Could you check a few things on this model? Use its own coordinates, in mm. A direction names the side the tool comes from. Coordinates: 2 decimals unless noted, no trailing zeros. Order: outer loops, then holes, each group sorted by start corner. A loop starts at its lowest first (then second) coordinate and runs counter-clockwise, first axis right, second up. Notation, with made-up numbers: (88.25, 1.5) -> (117.25, 1.5) arc R18 cw to (117.25, 26.5) -> close; hole circle Ø1 at (11.5, -31). An arc over 180 degrees is marked (long way). Put each result on its own line as item: value. Start each with the question number.
Q1. Will these pins go through, and if not, where does the flat tip stop? pin 1 (5 mm diameter, centred on x = -19, y = 8.5, fed in from +Z); pin 2 (8 mm diameter, centred on x = 20.5, y = 41.5, fed in from -Z); pin 3 (2.5 mm diameter, centred on x = -7.5, y = 60, fed in from +Z).
Q2. For faces 1 (the face through (18, 45, 25)), 2 (the face through (-0.6, 2, 9.2)), 3 (the face through (-18, 45, 25)), which set-ups out of +Z, -Z, +X, -X, +Y, -Y let a thin tool reach every point of the face, with its end or its side?
Q3. We'd pull the mould along Y, two halves only. Please class faces 4 (the face through (0, 48, 20)), 5 (the face through (-14.418, 10.058, -45.783)), 6 (the face through (21.01, 22.85, 25.04)): +Y half, -Y half, draft (parallel to the pull), parting line (faces both ways), or undercut.
Q4. Please list where these lines run through material, in increasing order: line 1 along Y through (x, z) = (17.5, -14.5); line 2 along Z through (x, y) = (-31, 4.5); line 3 along X through (y, z) = (16, -6).
Q5. If we section it at A-A (y = 48): Please give me the cut outline in (x, z), and give its area (3 significant figures).
from build123d import *

# Parameters (mm, degrees)
SKETCH2_R           = 1.15
SKETCH2_R_2         = 5
CUT_EXTRUDE1_DEPTH  = 74.484692283
BOSS_EXTRUDE1_START = 20
SKETCH6_R           = 5
SKETCH6_R_2         = 1
BOSS_EXTRUDE1_DEPTH = 10
FILLET1_R           = 10
CHAMFER1_SIZE       = 2


with BuildPart() as part:
    # Sketch1 → Revolve1 (revolve)
    with BuildSketch(Plane.XY, mode=Mode.PRIVATE) as revolve1_sk:
        Polygon((45, 0), (50, 5), (50, 15), (45, 20), (5, 20), (5, 0), align=None)
        Polygon((9, 2), (44.171572875, 2), (48, 5.828427125), (48, 14.171572875), (44.171572875, 18), (9, 18), align=None, mode=Mode.SUBTRACT)
    revolve(revolve1_sk.sketch.rotate(Axis((0, -3.9, 0), (0, 1, 0)), 90), axis=Axis((0, -3.9, 0), (0, 1, 0)))

    # Sketch2 → Cut-Extrude1 (cut, through all)
    with BuildSketch(Plane.XZ):
        with Locations(Location((7.5, 0, 0), (0, 0, 270))):
            Circle(SKETCH2_R)
        with Locations(Location((0, 7.5, 0), (0, 0, 270))):
            Circle(SKETCH2_R)
        with Locations(Location((-7.5, 0, 0), (0, 0, 270))):
            Circle(SKETCH2_R)
        with Locations(Location((0, -7.5, 0), (0, 0, 270))):
            Circle(SKETCH2_R)
        with Locations(Location((0, 0, 0), (0, 0, 270))):
            Circle(SKETCH2_R_2)
    extrude(amount=-CUT_EXTRUDE1_DEPTH, mode=Mode.SUBTRACT)

    # Sketch6 → Boss-Extrude1 (add)
    with BuildSketch(Plane.XY.offset(BOSS_EXTRUDE1_START)):
        with BuildLine():
            Line((18, 60), (18, 20))
            Line((18, 20), (-18, 20))
            Line((-18, 20), (-18, 60))
            ThreePointArc((-18, 60), (0, 78), (18, 60))
        make_face()
        with Locations((0, 60)):
            Circle(SKETCH6_R, mode=Mode.SUBTRACT)
        with Locations((0, 52.5)):
            Circle(SKETCH6_R_2, mode=Mode.SUBTRACT)
        with Locations((7.5, 60)):
            Circle(SKETCH6_R_2, mode=Mode.SUBTRACT)
        with Locations((0, 67.5)):
            Circle(SKETCH6_R_2, mode=Mode.SUBTRACT)
        with Locations((-7.5, 60)):
            Circle(SKETCH6_R_2, mode=Mode.SUBTRACT)
    extrude(amount=BOSS_EXTRUDE1_DEPTH)

    # Fillet1
    fillet1_edges = [part.edges().sort_by_distance(p)[0] for p in [
        (-18, 20, 25),
        (18, 20, 25),
    ]]
    fillet(fillet1_edges, radius=FILLET1_R)

    # Chamfer1
    # the kernel refuses this chamfer: 2 mm, written as the material it takes off along each edge
    with BuildSketch(Plane(origin=(0, 60, 30), x_dir=(-1, 0, 0), z_dir=(0, -1, 0))) as chamfer1_piece_1:
        Polygon((18, CHAMFER1_SIZE), (18 - CHAMFER1_SIZE, 0), (18, 0), align=None)
    revolve(axis=Axis((0, 60, 30), (0, 0, -1)), revolution_arc=180, mode=Mode.SUBTRACT)
    with BuildSketch(Plane(origin=(-18, 30, 30), x_dir=(-0.027495876610585647, 0, -0.9996219169112968), z_dir=(0, 1, 0)), Plane(origin=(18, 60, 30), x_dir=(0.027495876610585647, 0, -0.9996219169112968), z_dir=(0, -1, 0))) as chamfer1_piece_2:
        Polygon((CHAMFER1_SIZE * 0.999621916911, -CHAMFER1_SIZE * 0.0274958766106), (-CHAMFER1_SIZE * 0.0274958766106, -CHAMFER1_SIZE * 0.999621916911), (0, 0), align=None)
    extrude(amount=30, mode=Mode.SUBTRACT)
    with BuildSketch(Plane(origin=(0, 60, 20), x_dir=(-1, 0, 0), z_dir=(0, -1, 0))) as chamfer1_piece_3:
        Polygon((18, -CHAMFER1_SIZE), (18 - CHAMFER1_SIZE, 0), (18, 0), align=None)
    revolve(axis=Axis((0, 60, 20), (0, 0, -1)), revolution_arc=180, mode=Mode.SUBTRACT)
    with BuildSketch(Plane(origin=(-18, 30, 20), x_dir=(-0.027495876610585647, 0, 0.9996219169112968), z_dir=(0, 1, 0)), Plane(origin=(18, 60, 20), x_dir=(0.027495876610585647, 0, 0.9996219169112968), z_dir=(0, -1, 0))) as chamfer1_piece_4:
        Polygon((CHAMFER1_SIZE * 0.999621916911, CHAMFER1_SIZE * 0.0274958766106), (-CHAMFER1_SIZE * 0.0274958766106, CHAMFER1_SIZE * 0.999621916911), (0, 0), align=None)
    extrude(amount=30, mode=Mode.SUBTRACT)
    with BuildSketch(Plane(origin=(-28, 30, 20), x_dir=(-0.49213725734726604, -0.8705176160944192, 0), z_dir=(-0.8705176160944192, 0.49213725734726604, 0))) as chamfer1_piece_5_section:
        Polygon((10, CHAMFER1_SIZE), (10 + CHAMFER1_SIZE, 0), (10, 0), align=None)
    chamfer1_piece_5 = revolve(axis=Axis((-28, 30, 20), (0, 0, 1)), revolution_arc=119.481154356, mode=Mode.PRIVATE)
    chamfer1_piece_5 = split(chamfer1_piece_5, bisect_by=Plane(origin=(-20.846294556, 20, 20.72247208), z_dir=(0, 1, 0)), keep=Keep.TOP, mode=Mode.PRIVATE)
    add(chamfer1_piece_5, mode=Mode.SUBTRACT)
    with BuildSketch(Plane(origin=(-28, 30, 30), x_dir=(-0.49213725734726604, -0.8705176160944192, 0), z_dir=(-0.8705176160944192, 0.49213725734726604, 0))) as chamfer1_piece_6_section:
        Polygon((10, -CHAMFER1_SIZE), (10 + CHAMFER1_SIZE, 0), (10, 0), align=None)
    chamfer1_piece_6 = revolve(axis=Axis((-28, 30, 30), (0, 0, 1)), revolution_arc=119.481154356, mode=Mode.PRIVATE)
    chamfer1_piece_6 = split(chamfer1_piece_6, bisect_by=Plane(origin=(-20.846294556, 20, 29.27752792), z_dir=(0, 1, 0)), keep=Keep.TOP, mode=Mode.PRIVATE)
    add(chamfer1_piece_6, mode=Mode.SUBTRACT)
    with BuildSketch(Plane(origin=(28, 30, 20), x_dir=(0.49213725734726604, -0.8705176160944192, 0), z_dir=(0.8705176160944192, 0.49213725734726604, 0))) as chamfer1_piece_7_section:
        Polygon((10, -CHAMFER1_SIZE), (10 + CHAMFER1_SIZE, 0), (10, 0), align=None)
    chamfer1_piece_7 = revolve(axis=Axis((28, 30, 20), (0, 0, -1)), revolution_arc=119.481154356, mode=Mode.PRIVATE)
    chamfer1_piece_7 = split(chamfer1_piece_7, bisect_by=Plane(origin=(20.846294556, 20, 20.72247208), z_dir=(0, 1, 0)), keep=Keep.TOP, mode=Mode.PRIVATE)
    add(chamfer1_piece_7, mode=Mode.SUBTRACT)
    with BuildSketch(Plane(origin=(28, 30, 30), x_dir=(0.49213725734726604, -0.8705176160944192, 0), z_dir=(0.8705176160944192, 0.49213725734726604, 0))) as chamfer1_piece_8_section:
        Polygon((10 + CHAMFER1_SIZE, 0), (10, CHAMFER1_SIZE), (10, 0), align=None)
    chamfer1_piece_8 = revolve(axis=Axis((28, 30, 30), (0, 0, -1)), revolution_arc=119.481154356, mode=Mode.PRIVATE)
    chamfer1_piece_8 = split(chamfer1_piece_8, bisect_by=Plane(origin=(20.846294556, 20, 29.27752792), z_dir=(0, 1, 0)), keep=Keep.TOP, mode=Mode.PRIVATE)
    add(chamfer1_piece_8, mode=Mode.SUBTRACT)


solid = part.part
The answers:
1. pin 1: z = 47.2
1. pin 2: z = 20.5
1. pin 3: z = 30
2. face 1: +Z, -Z, +X, +Y
2. face 2: none
2. face 3: +Z, -Z, -X, +Y
3. face 4: draft
3. face 5: undercut
3. face 6: +Y half
4. line 1: 0 to 2, 18 to 20
4. line 2: -38.59 to -34.89, 34.89 to 38.59
4. line 3: -48.63 to -45.78, -6.71 to 6.71, 45.78 to 48.63
5. outline: (-18, 22) -> (-16, 20) -> (16, 20) -> (18, 22) -> (18, 28) -> (16, 30) -> (-16, 30) -> (-18, 28) -> close
5. area: 352 mm^2
